Autodesk Inventor part; units mm, degrees
ref_plane "YZ Plane" through (0, 0, 0) normal (1, 0, 0) x (0, 1, 0)
ref_plane "XZ Plane" through (0, 0, 0) normal (0, 1, 0) x (-1, 0, 0)
ref_plane "XY Plane" through (0, 0, 0) normal (0, 0, 1) x (1, 0, 0)
sketch "スケッチ1" plane through (0, 0, 0) normal (0, 0, 1) x (1, 0, 0)
  line L0 (-3.5, 3.25) -> (3.5, 3.25)
  line L1 (3.5, 3.25) -> (3.5, -3.25)
  line L2 (3.5, -3.25) -> (-3.5, -3.25)
  line L3 (-3.5, -3.25) -> (-3.5, 3.25)
  line L4 (-3.5, 3.25) -> (3.5, -3.25) construction
  line L5 (3.5, 3.25) -> (-3.5, -3.25) construction
  line L6 (-2.5, 3.25) -> (-2.5, -3.25) construction
  line L7 (2.5, 3.25) -> (2.5, -3.25) construction
  line L8 (0, 0) -> (0, 0.4773) construction
  line L9 (0, 0) -> (0.5273, 0) construction
  line L10 (-1.5, 1.5) -> (1.5, 1.5)
  line L11 (1.5, 1.5) -> (1.5, -1.5)
  line L12 (1.5, -1.5) -> (-1.5, -1.5)
  line L13 (-1.5, -1.5) -> (-1.5, 1.5)
  line L14 (-1.5, 1.5) -> (1.5, -1.5) construction
  line L15 (1.5, 1.5) -> (-1.5, -1.5) construction
  circle A0 centre (0, 0) radius 0.8
  dimension "d0" = 7
  dimension "d1" = 6.5
  dimension "d2" = 5
  dimension "d22" = 3
  dimension "d23" = 3
  dimension "d24" = 1.6
extrude "押し出し1" add sketch "スケッチ1" along normal blind 13.5 contours L0 L1 L2 L3 | L10 L11 L12 L13 | A0
ref_plane "作業平面1" through (-3.5, -3.25, 0) normal (0, -1, 0) x (1, 0, 0)
sketch "スケッチ2" plane through (-3.5, -3.25, 0) normal (0, -1, 0) x (1, 0, 0)
  line L0 (0, 0) -> (7, 0)
  line L1 (7, 0) -> (7, 13.5)
  line L2 (0, 13.5) -> (7, 13.5)
  line L3 (0, 0) -> (0, 13.5)
  line L4 (0, 0) -> (0, 13.5)
  line L5 (7, 0) -> (7, 13.5)
  line L6 (0, 0) -> (7, 0)
  line L7 (0, 0) -> (0, 13.5)
  line L8 (0, 1.5) -> (7, 1.5) construction
  line L9 (0, 6.5) -> (7, 6.5) construction
  line L10 (7, 0) -> (7, 13.5)
  line L11 (0, 6.5) -> (7, 1.5) construction
  line L12 (7, 6.5) -> (0, 1.5) construction
  circle A0 centre (3.5, 4) radius 2.5
  line L13 (0, 7) -> (7, 7)
  line L14 (0, 7) -> (0, 13.5)
  line L15 (0, 13.5) -> (7, 13.5)
  line L16 (7, 13.5) -> (7, 7)
  line L17 (7, 13.5) -> (0, 13.5)
  point P0 (3.5, 0)
  point P1 (0, 7)
  point P2 (7, 7)
  dimension "d8" = 1.5
  dimension "d9" = 5
  dimension "d10" = 5
  dimension "d11" = 0.5
extrude "押し出し2" add sketch "スケッチ2" along normal blind 3 contours L3 L2 L1 L13
ref_plane "作業平面2" through (-3.5, -6.25, 0) normal (0, -1, 0) x (1, 0, 0)
sketch "スケッチ3" plane through (-3.5, -6.25, 0) normal (0, -1, 0) x (1, 0, 0)
  line L0 (7, 7) -> (7, 13.5)
  line L1 (7, 13.5) -> (0, 13.5)
  line L2 (0, 13.5) -> (0, 7)
  line L3 (0, 7) -> (7, 7)
  line L4 (0, 0) -> (0, 13.5)
  line L5 (7, 7) -> (7, 13.5)
  line L6 (0, 7) -> (7, 7)
  line L7 (0, 7.5) -> (7, 7.5) construction
  line L8 (7, 0) -> (7, 13.5)
  line L9 (0, 12.5) -> (7, 12.5) construction
  line L10 (0, 12.5) -> (7, 7.5) construction
  line L11 (7, 12.5) -> (0, 7.5) construction
  circle A0 centre (3.5, 10) radius 2.5
  point P0 (3.5, 0)
  dimension "d15" = 0.5
  dimension "d16" = 1
  dimension "d17" = 5
extrude "押し出し3" cut sketch "スケッチ3" against normal up to surface (9.5 mm away) contours A0
extrude "押し出し4" cut sketch "スケッチ2" against normal blind 10 contours A0
extrude "押し出し5" add sketch "スケッチ1" against normal blind 2.9 contours L10 L11 L12 L13 | A0
chamfer "面取り1" distance 1.5 angle 45 2 edges at (3.5, -1.5, 13.5) (-3.5, -1.5, 13.5)
properties part number "sensorholder_2"
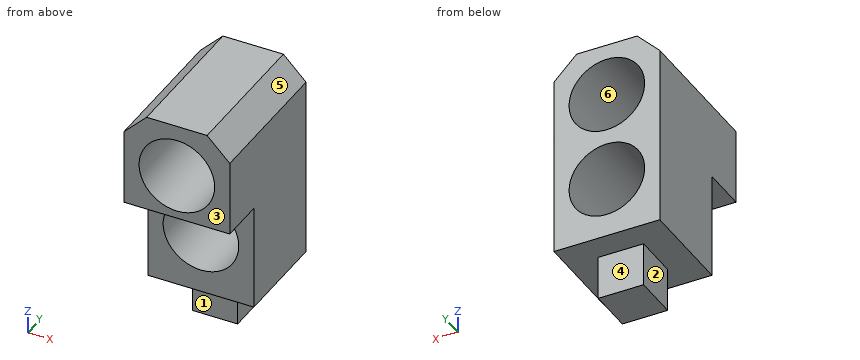
Could you check a few things on this model? Use its own coordinates, in mm. Face numbers are marked on the shaded views. A direction names the side the tool comes from. Give positions to 0.01 mm unless a question says otherwise; leave off trailing zeros. Order: outer loops, then holes, each group sorted by start corner. A loop starts at its lowest first (then second) coordinate and runs counter-clockwise, first axis right, second up. Notation, with made-up numbers: (78, -19.75) - (111, -19.75) arc R14 ccw to (111, -15.75) - close; hole circle Ø4 at (44, 40). An arc over 180 degrees is marked (long way). Return JSON: item names as keys, results as strings. Group by question number.
Q1. Suppose I cut it at A-A, the plane z = 6. Please give me the cut outline in (x, y).
Q2. Will these pins go through, and if not, where does the flat tip stop? pin 1 Ø1.4 at (x, z) = (-0.5, -1.5) entering from -Y; pin 2 Ø1.4 at (x, z) = (-0.5, -1.5) entering from +Y; pin 3 Ø0.9 at (y, z) = (-0.5, -1) entering from +X.
Q3. Please list where these lines run through material, in increasing order: line 1 along Z through (x, y) = (0, 0.25); line 2 along Z through (x, y) = (0, 2.25); line 3 along X through (y, z) = (-5.25, 11.5). Write a range as [from, to].
Q4. Which directions (+Z, -Z, +X, -X, +Y, -Y) give clear straight access to the entire face, cutting with the end or side of a thin tool? Please do the marked faces 1, 2 and 3.
Q5. Thinking about a two-plate mould opening in Z: for the marked faces 4, 5 and 6, which applies, pulls with the +Z half, pulls with the -Z half, needs draft (parallel to the pull), parting line crosses it, or undercut?
Q6. Suppose I cut it at C-C, the plane x = 0.75. Please give me the cut outline in (y, z), and give its area (3 significant figures).
Q7. Suppose I cut it at D-D, the plane z = 4. Please give me the cut outline in (x, y).
Q8. Suppose I cut it at B-B, the plane y = 1.25. Please give me the cut outline in (x, z).
Resolved:
{
 "1": {"outline": "(-3.5, -3.25) - (-1.5, -3.25) - (-1.5, 3.25) - (-3.5, 3.25) - close; (1.5, -3.25) - (3.5, -3.25) - (3.5, 3.25) - (1.5, 3.25) - close"},
 "2": {"pin 1": "stops at y = -1.5", "pin 2": "stops at y = 1.5", "pin 3": "stops at x = 1.5"},
 "3": {"line 1": "z = [-2.9, 1.5], [6.5, 7.5], [12.5, 13.5]", "line 2": "z = [0, 1.5], [6.5, 7.5], [12.5, 13.5]", "line 3": "x = [-3.5, -2], [2, 3.5]"},
 "4": {"face 1": "-Z, +X, -X, -Y", "face 2": "-Z, -X, +Y, -Y", "face 3": "+Z, -Z, +X, -X, -Y"},
 "5": {"face 4": "needs draft", "face 5": "pulls with the +Z half", "face 6": "undercut"},
 "6": {"outline": "(-6.25, 7) - (-3.25, 7) - (-3.25, 6.38) - (3.25, 6.38) - (3.25, 7.62) - (-6.25, 7.62) - close; (-6.25, 12.38) - (3.25, 12.38) - (3.25, 13.5) - (-6.25, 13.5) - close; (-3.25, 0) - (-1.5, 0) - (-1.5, -2.9) - (1.5, -2.9) - (1.5, 0) - (3.25, 0) - (3.25, 1.62) - (-3.25, 1.62) - close", "area": "39.6 mm2"},
 "7": {"outline": "(-3.5, -3.25) - (-2.5, -3.25) - (-2.5, 3.25) - (-3.5, 3.25) - close; (2.5, -3.25) - (3.5, -3.25) - (3.5, 3.25) - (2.5, 3.25) - close"},
 "8": {"outline": "(-3.5, 0) - (-1.5, 0) - (-1.5, -2.9) - (1.5, -2.9) - (1.5, 0) - (3.5, 0) - (3.5, 12) - (2, 13.5) - (-2, 13.5) - (-3.5, 12) - close; hole circle Ø5 at (0, 4); hole circle Ø5 at (0, 10)"}
}
